Input: part model. Units: mm. Frame: model coordinates. A direction names the side the tool comes from. Give positions to 0.01 mm unless a question says otherwise; leave off trailing zeros. Order: outer loops, then holes, each group sorted by start corner. A loop starts at its lowest first (then second) coordinate and runs counter-clockwise, first axis right, second up. Notation, with made-up numbers: (6, -8) - (20, -8) arc R24 cw to (20, 20) - close; hole circle Ø4 at (65, 29.5). An arc over 180 degrees is marked (long way). Use a Markdown table: item, result.
from build123d import *

# Parameters (mm, degrees)
SKETCH_1_R         = 4.9
EXTRUDE_1_DEPTH    = 15
HOLE_WIZARD_M4_1_D = 3.3
CHAMFER_1_SIZE     = 1
SKETCH_6_R         = 2.1
EXTRUDE_2_DEPTH    = 3


with BuildPart() as part:
    # 草图1 → 凸台-拉伸1 (new body)
    with BuildSketch(Plane(origin=(0, 0, 0), x_dir=(1, 0, 0), z_dir=(0, 1, 0))):
        with Locations(Location((0, 0, 0), (0, 0, 270))):
            Circle(SKETCH_1_R)
    extrude(amount=EXTRUDE_1_DEPTH)

    # M4 螺纹孔1 (through all)
    with Locations(Plane(origin=(4.9, 0, 0), x_dir=(0, 0, -1), z_dir=(1, 0, 0))):
        with Locations((0, 5)):
            Hole(HOLE_WIZARD_M4_1_D / 2)

    # 倒角1
    chamfer_1_edges = [part.edges().sort_by_distance(p)[0] for p in [
        (0, 0, -4.9),
    ]]
    chamfer(chamfer_1_edges, length=CHAMFER_1_SIZE)

    # 草图6 → 凸台-拉伸2 (add)
    with BuildSketch(Plane(origin=(0, 15, 0), x_dir=(1, 0, 0), z_dir=(0, 1, 0))):
        with BuildLine():
            Line((-12.5, 7.5), (12.5, 7.5))
            ThreePointArc((12.5, 7.5), (20, 0), (12.5, -7.5))
            Line((12.5, -7.5), (-12.5, -7.5))
            ThreePointArc((-12.5, -7.5), (-20, 0), (-12.5, 7.5))
        make_face()
        with Locations(Location((-12.5, 0, 0), (0, 0, 270))):
            Circle(SKETCH_6_R, mode=Mode.SUBTRACT)
        with Locations(Location((12.5, 0, 0), (0, 0, 270))):
            Circle(SKETCH_6_R, mode=Mode.SUBTRACT)
    extrude(amount=-EXTRUDE_2_DEPTH)


solid = part.part
1. Set-up query: faces 1 (the face through (-4.347, 6.423, 2.261)), 2 (the face through (0, 14, 7.5)). Return all of +Z, -Z, +X, -X, +Y, -Y with unobstructed straight access to the full face (end or side cutting, diameter ignored); none if empty.
Response:
| item | result |
|---|---|
| face 1 | -Y |
| face 2 | +Z, +X, -X, +Y, -Y |
2. Section query A-A (z = 0). Return loops of the section in (x, y).
Response:
| item | result |
|---|---|
| outline | (-20, 12) - (-14.6, 12) - (-14.6, 15) - (-20, 15) - close; (-10.4, 12) - (-4.9, 12) - (-4.9, 6.65) - (4.9, 6.65) - (4.9, 12) - (10.4, 12) - (10.4, 15) - (-10.4, 15) - close; (-4.9, 1) - (-3.9, 0) - (3.9, 0) - (4.9, 1) - (4.9, 3.35) - (-4.9, 3.35) - close; (14.6, 12) - (20, 12) - (20, 15) - (14.6, 15) - close |
3. Section query D-D (y = 14). Return loops of the section in (x, z), then the cut area to 3 significant figures.
Response:
| item | result |
|---|---|
| outline | (-12.5, -7.5) - (12.5, -7.5) arc R7.5 ccw to (12.5, 7.5) - (-12.5, 7.5) arc R7.5 ccw to start; hole circle Ø4.2 at (-12.5, 0); hole circle Ø4.2 at (12.5, 0) |
| area | 524 mm^2 |
4. Mould query, pull axis X, two halves, no side actions, for faces 3 (the face through (-0.1, 3.4, -0.4)), 4 (the face through (14.27, 13.52, 1.13)), 5 (the face through (20, 14, 0)). Classes: pulls with the +X half, pulls with the -X half, needs draft (parallel to the pull), parting line crosses it, or undercut.
Response:
| item | result |
|---|---|
| face 3 | needs draft |
| face 4 | undercut |
| face 5 | pulls with the +X half |
5. Pin query (flat end, axial travel): pin 1 (5.5 mm diameter, centred on y = 5, z = 0, fed in from -X); pin 2 (8 mm diameter, centred on y = 9, z = 3, fed in from +X); pin 3 (5 mm diameter, centred on x = -15.5, z = 0.5, fed in from -Y). Return the tip coordinate at first contact, or that it passes through.
Response:
| item | result |
|---|---|
| pin 1 | stops at x = -4.9 |
| pin 2 | stops at x = 19.99 |
| pin 3 | stops at y = 12 |
6. Section query B-B (x = -11.5). Return loops of the section in (y, z), then the cut area to 3 significant figures.
Response:
| item | result |
|---|---|
| outline | (12, -7.5) - (15, -7.5) - (15, -1.85) - (12, -1.85) - close; (12, 1.85) - (15, 1.85) - (15, 7.5) - (12, 7.5) - close |
| area | 33.9 mm^2 |
7. Material intervals for line 1 along X through (y, z) = (14.15, 0); line 2 along X through (y, z) = (14.25, 1.25); line 3 along Y through (x, z) = (15.5, 3), sorted ascending.
Response:
| item | result |
|---|---|
| line 1 | x = -20 to -14.6, -10.4 to 10.4, 14.6 to 20 |
| line 2 | x = -19.9 to -14.19, -10.81 to 10.81, 14.19 to 19.9 |
| line 3 | y = 12 to 15 |
8. Section query C-C (x = 0). Return loops of the section in (y, z), then the cut area to 3 significant figures.
Response:
| item | result |
|---|---|
| outline | (0, -3.9) - (1, -4.9) - (12, -4.9) - (12, -7.5) - (15, -7.5) - (15, 7.5) - (12, 7.5) - (12, 4.9) - (1, 4.9) - (0, 3.9) - close; hole circle Ø3.3 at (5, 0) |
| area | 153 mm^2 |
